For this review, take the finished solid that the model builds, in its own axes (mm). Round coordinates to 2 decimals unless told otherwise and drop trailing zeros. Loops run counter-clockwise (first coordinate to the right, second up) from the corner with the lowest first, then second, coordinate; pieces in that order, holes last. Notation, with made-up numbers: (26, 37) -> (83, 37) arc R9 ccw to (83, 44) -> close; hole circle Ø8 at (-13, 49). An arc over 180 degrees is marked (long way). One line per question, with ' | ' between items. Start each with the question number.
1. For pin 1 Ø1 at (x, y) = (0.5, 2.5) entering from -Z; pin 2 Ø1.5 at (x, z) = (2, -1) entering from +Y, all flat-tipped, find the tip position at first contact; note any pin that passes through.
2. Wall thickness on line 1 along Y through (x, z) = (1.2, 0); line 2 along X through (y, z) = (-4.5, 7.25); line 3 along X through (y, z) = (-1.5, 8): over which ranges is each line inside the solid? List them lowest first.
3. Draft analysis for pull direction X (two halves, no side actions). For faces 1 (the face through (2.5, 2, 0)), 2 (the face through (-2.5, 2, 0)), 3 (the face through (-0.02, 7.81, -1.73)), state which applies: pulls with the +X half, pulls with the -X half, needs draft (parallel to the pull), parting line crosses it, or undercut.
4. Consider section C-C (x = 0.65). Write out the cut boundary in (y, z), and give its area (3 significant figures).
```python
from build123d import *

# Parameters (mm, degrees)
FILLET1_R = 0.5


with BuildPart() as part:
    # Sketch1 → Revolve1 (revolve)
    with BuildSketch(Plane.XY, mode=Mode.PRIVATE) as revolve1_sk:
        with BuildLine():
            Line((-2.5, 1.5), (2.5, 1.5))
            Line((2.5, 1.5), (2.5, 9))
            Line((2.5, 9), (1.75, 9))
            Line((1.75, 9), (1.75, 8.5))
            ThreePointArc((1.75, 8.5), (1.603553391, 8.146446609), (1.25, 8))
            Line((1.25, 8), (-1.25, 8))
            ThreePointArc((-1.25, 8), (-1.603553391, 8.146446609), (-1.75, 8.5))
            Line((-1.75, 8.5), (-1.75, 9))
            Line((-1.75, 9), (-2.5, 9))
            Line((-2.5, 9), (-2.5, 1.5))
        make_face()
    revolve(revolve1_sk.sketch.rotate(Axis((0, 0, 0), (1, 0, 0)), 90), axis=Axis((0, 0, 0), (1, 0, 0)))

    # Fillet1
    fillet1_edges = [part.edges().sort_by_distance(p)[0] for p in [
        (1.75, 0, -9),
        (-1.75, 0, -9),
    ]]
    fillet(fillet1_edges, radius=FILLET1_R - 0.0001)  # a hair under: the kernel refuses the full size


solid = part.part
```
Answer block:
1) pin 1: stops at z = -7.75 | pin 2: stops at y = 9
2) line 1: y = -8 to -1.5, 1.5 to 8 | line 2: x = -2.5 to -1.75, 1.75 to 2.5 | line 3: x = -2.5 to -1.6, 1.6 to 2.5
3) face 1: pulls with the +X half | face 2: pulls with the -X half | face 3: undercut
4) outline: circle Ø16 at (0, 0); hole circle Ø3 at (0, 0) | area: 194 mm2
